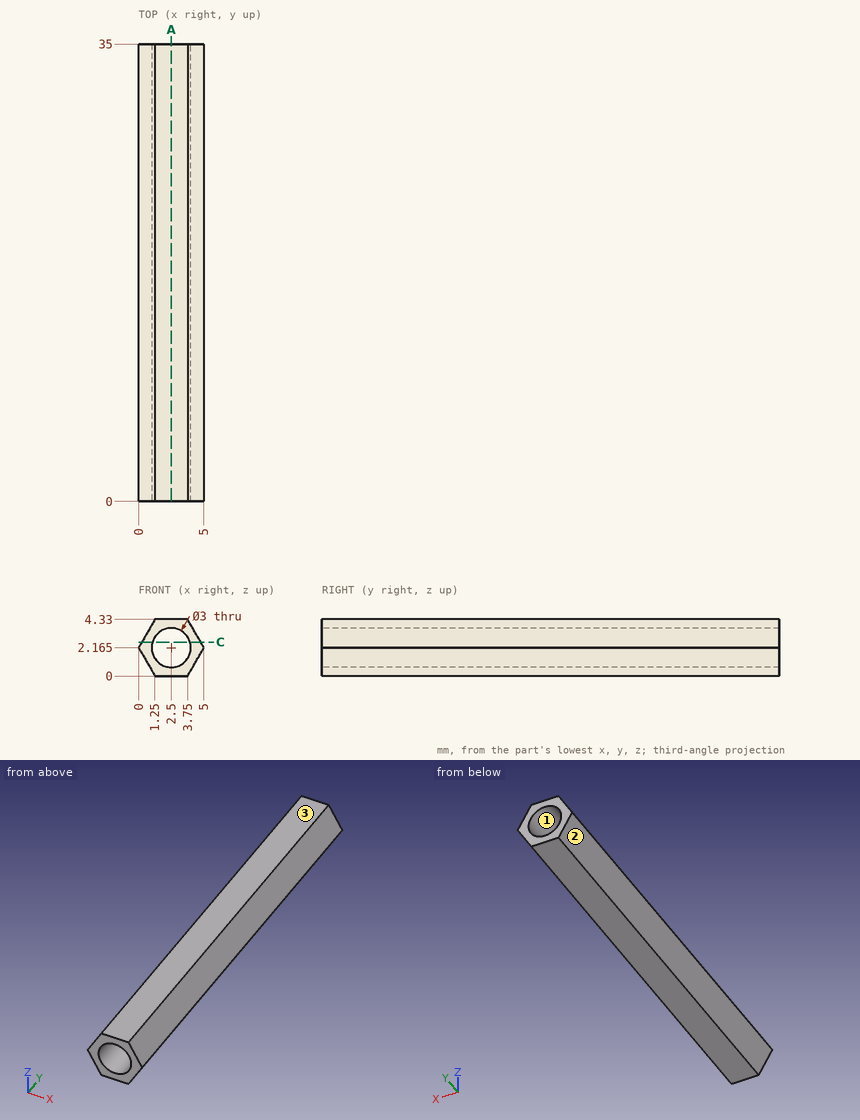
Could you check a few things on this drawing? It's one solid part, dimensions in mm from its lowest x, y, z. Round coordinates to 2 decimals unless told otherwise and drop trailing zeros. Write each loop counter-clockwise with the first axis right and the second up, starting at its lowest first coordinate (ties: lowest second). Pieces come first, ordered by that corner, then holes. Notation, with made-up numbers: (-36.5, -21) -> (-7.5, -21) arc R16 cw to (-7.5, -6) -> close; hole circle Ø8 at (-34, 28.25). An arc over 180 degrees is marked (long way). One line per item, written item: value.
1) If I drill on line 1 (Z direction, x = 2.5, y = 18) (1 decimal); line 2 (X direction, y = 23.5, z = 3.3) (1 decimal); line 3 (X direction, y = 21.5, z = 1.6), over which ranges is the centre line in solid material (lowest first)? Write a range as [from, to].
Filled sheet:
line 1: z = [0, 0.7], [3.7, 4.3]
line 2: x = [0.7, 1.5], [3.5, 4.3]
line 3: x = [0.33, 1.11], [3.89, 4.67]
2) We'd pull the mould along Z, two halves only. Please class the marked faces 1, 2 and 3: released by +Z, released by -Z, zero draft, split by the parting line, or undercut.
Filled sheet:
face 1: undercut
face 2: released by -Z
face 3: released by +Z
3) Suppose I cut it at A-A on x = 2.5. List the corners of the cut face in (y, z) for me (1 decimal).
Filled sheet:
outline: (0, 0) -> (35, 0) -> (35, 0.7) -> (0, 0.7) -> close; (0, 3.7) -> (35, 3.7) -> (35, 4.3) -> (0, 4.3) -> close
4) Suppose I cut it at C-C on z = 2.6. List the corners of the cut face in (x, y) for me.
Filled sheet:
outline: (0.25, 0) -> (1.06, 0) -> (1.06, 35) -> (0.25, 35) -> close; (3.94, 0) -> (4.75, 0) -> (4.75, 35) -> (3.94, 35) -> close
